Read the model definition and answer for the solid it produces. Units are mm, in the model's axes. A direction names the side the tool comes from. Coordinates: 2 decimals unless noted, no trailing zeros. Write each loop counter-clockwise with the first axis right and the second up, starting at its lowest first coordinate (ties: lowest second). Pieces come first, ordered by that corner, then holes.
(1) Which of the six approach directions +Z, -Z, +X, -X, +Y, -Y give full straight-line access (tool end or side, diameter ignored) to faces 1 (the cylindrical face through (7.667, 10.16, 9.999)), 2 (the flat face through (11.3, 14.4, 1.9)), 3 (the cylindrical face through (-3.034, 2.941, -9.634))?
(2) The part is cut by section A-A, the plane y = 20. Determine the outline of the cut face in (x, z).
(3) Straight lines are drawn through the part: line 1 along Y through (x, z) = (2.5, -11.5); line 2 along Y through (x, z) = (1.5, 5.75); line 3 along Z through (x, y) = (3, 24.5). For each, find the intervals that lie inside material, in ascending order.
(4) The part is cut by section B-B, the plane y = 8. Determine the outline of the cut face in (x, z), and give its area (3 significant figures).
(5) Given pin 1 (8 mm diameter, centred on x = 6.5, y = 16.5, fed in from -Z); pin 2 (3 mm diameter, centred on x = 6, y = 25.5, fed in from +Z); pin 3 (3 mm diameter, centred on x = -2, y = 31, fed in from -Z), each flat-ended and moving along its own axis, determine where each tip first touches the part or whether it passes through.
Autodesk Inventor part; units mm, degrees
ref_plane "YZ Plane" through (0, 0, 0) normal (1, 0, 0) x (0, 1, 0)
ref_plane "XZ Plane" through (0, 0, 0) normal (0, 1, 0) x (-1, 0, 0)
ref_plane "XY Plane" through (0, 0, 0) normal (0, 0, 1) x (1, 0, 0)
sketch "Sketch1" plane through (0, 0, 0) normal (1, 0, 0) x (0, 1, 0)
  line L0 (0, 0) -> (0, -10.1)
  line L1 (0, -10.1) -> (5.8, -10.1)
  line L2 (5.8, -10.1) -> (5.8, -12.6)
  line L3 (5.8, -12.6) -> (14.4, -12.6)
  line L4 (14.4, -12.6) -> (14.4, -11.3)
  line L5 (14.4, -11.3) -> (30, -11.3)
  line L6 (30, -11.3) -> (37.55, -11.3)
  line L7 (37.55, -11.3) -> (37.55, -8.7)
  line L8 (37.55, -8.7) -> (30, -11.3)
  line L9 (37.55, -8.7) -> (39.2214, 0)
  line L10 (39.2214, 0) -> (0, 0)
  dimension "d0" = 10.1
  dimension "d1" = 5.8
  dimension "d2" = 90
  dimension "d3" = 2.5
  dimension "d4" = 90
  dimension "d5" = 8.6
  dimension "d6" = 1.3
  dimension "d7" = 90
  dimension "d8" = 15.6
  dimension "d9" = 7.55
  dimension "d10" = 2.6
revolve "Revolution1" add sketch "Sketch1" angle 360 about axis through (0, 39.2214, 0) along (0, -1, 0) contours L10 L9 L8 L5 L4 L3 L2 L1 L0
properties part number "30_CUBE_openSIM_ObjectiveLens_10x"
Computed:
1. face 1: +Y, -Y
1. face 2: +Y
1. face 3: -Y
2. outline: circle Ø22.6 at (0, 0)
3. line 1: y = 5.8 to 14.4
3. line 2: y = 0 to 38.08
3. line 3: z = -10.89 to 10.89
4. outline: circle Ø25.2 at (0, 0)
4. area: 499 mm2
5. pin 1: stops at z = -12.21
5. pin 2: stops at z = 10.37
5. pin 3: stops at z = -11.27
